The model under review builds one solid part; all positions refer to its coordinate system, in mm. Round coordinates to 2 decimals unless told otherwise and drop trailing zeros. Order: outer loops, then holes, each group sorted by start corner. A loop starts at its lowest first (then second) coordinate and runs counter-clockwise, first axis right, second up. Notation, with made-up numbers: (79.5, 48) -> (97.5, 48) arc R21 ccw to (97.5, 76) -> close; hole circle Ø3 at (31.25, 28). An arc over 180 degrees is marked (long way). Use a Markdown table: item, result. Add a question column.
```python
from build123d import *

# Parameters (mm, degrees)
F0_R          = 40.64
F0_R_2        = 39.37
F1_DEPTH      = 3.175
F2_R          = 1.5875
F4_DEPTH      = 40.641
F4_DEPTH_BACK = 49.77658
F3_R          = 1.5875
F5_DEPTH      = 40.6410001
F5_DEPTH_BACK = 44.7205


with BuildPart() as f1:
    # F0 (on Front) → F1 (new body, symmetric)
    with BuildSketch(Plane.XZ):
        Circle(F0_R)
        Circle(F0_R_2, mode=Mode.SUBTRACT)
    extrude(amount=F1_DEPTH, both=True)

    # F2 (on Top) → F4 (cut, two sides)
    with BuildSketch(Plane.XY) as f4_sk:
        Circle(F2_R)
    extrude(amount=-F4_DEPTH, mode=Mode.SUBTRACT)
    extrude(f4_sk.sketch, amount=F4_DEPTH_BACK, mode=Mode.SUBTRACT)

    # F3 (on Right) → F5 (cut, two sides)
    with BuildSketch(Plane.YZ) as f5_sk:
        Circle(F3_R)
    extrude(amount=-F5_DEPTH, mode=Mode.SUBTRACT)
    extrude(f5_sk.sketch, amount=F5_DEPTH_BACK, mode=Mode.SUBTRACT)


solid = f1.part
```
Q1. For pin 1 (2.5 mm diameter, centred on y = 0, z = 0, fed in from -X), flat-tipped, find the tip position at first contact; note if it passes through.
Q2. Draft analysis for pull direction Z (two halves, no side actions). For faces 1 (the face through (-0.34, -1.55, 39.98)), 2 (the face through (-5.291, -0.044, 40.294)), 3 (the face through (-31.24, 0.04, -23.96)), state which applies: released by +Z, released by -Z, zero draft, split by the parting line, or undercut.
Q3. Add section D-D, the plane x = -31. Give the boundary of the cut face in (y, z) (3 decimals).
Q4. Add section B-B, the plane x = 0. Give the boundary of the cut face in (y, z) (1 decimal), then the cut area to 3 significant figures.
Q5. Add section C-C, the plane z = 35.5. Give the boundary of the cut face in (x, y) (3 decimals).
Q6. Add section A-A, the plane z = 0. Give the boundary of the cut face in (x, y) (1 decimal).
Q7. To check wall thickness, follow line 1 along Z through (x, y) = (0, -1.75); line 2 along Y through (x, z) = (0, 40.3) (1 decimal); line 3 along X through (y, z) = (2, 30). State the ranges of each line that lie inside material, in increasing order.
Return value:
| question | item | result |
|---|---|---|
| 1 | pin 1 | through |
| 2 | face 1 | zero draft |
| 2 | face 2 | split by the parting line |
| 2 | face 3 | undercut |
| 3 | outline | (-3.175, -26.279) -> (3.175, -26.279) -> (3.175, -24.269) -> (-3.175, -24.269) -> close; (-3.175, 24.269) -> (3.175, 24.269) -> (3.175, 26.279) -> (-3.175, 26.279) -> close |
| 4 | outline | (-3.2, -40.6) -> (-1.6, -40.6) -> (-1.6, -39.4) -> (-3.2, -39.4) -> close; (-3.2, 39.4) -> (-1.6, 39.4) -> (-1.6, 40.6) -> (-3.2, 40.6) -> close; (1.6, -40.6) -> (3.2, -40.6) -> (3.2, -39.4) -> (1.6, -39.4) -> close; (1.6, 39.4) -> (3.2, 39.4) -> (3.2, 40.6) -> (1.6, 40.6) -> close |
| 4 | area | 8.06 mm² |
| 5 | outline | (-19.783, -3.175) -> (-17.022, -3.175) -> (-17.022, 3.175) -> (-19.783, 3.175) -> close; (17.022, -3.175) -> (19.783, -3.175) -> (19.783, 3.175) -> (17.022, 3.175) -> close |
| 6 | outline | (-40.6, -3.2) -> (-39.4, -3.2) -> (-39.4, -1.6) -> (-40.6, -1.6) -> close; (-40.6, 1.6) -> (-39.4, 1.6) -> (-39.4, 3.2) -> (-40.6, 3.2) -> close; (39.4, -3.2) -> (40.6, -3.2) -> (40.6, -1.6) -> (39.4, -1.6) -> close; (39.4, 1.6) -> (40.6, 1.6) -> (40.6, 3.2) -> (39.4, 3.2) -> close |
| 7 | line 1 | -40.64 to -39.37, 39.37 to 40.64 |
| 7 | line 2 | -3.2 to -1.6, 1.6 to 3.2 |
| 7 | line 3 | -27.42 to -25.5, 25.5 to 27.42 |
